Drawing for the job (mm, zero at the part's lowest x, y, z). A direction names the side the tool comes from. Give positions to 0.01 mm unless a question says otherwise; leave off trailing zeros. Loops run counter-clockwise (first coordinate to the right, second up) from the corner with the lowest first, then second, coordinate; pieces in that order, holes last. Notation, with made-up numbers: (-22.75, -4.75) - (5.25, -4.75) arc R7 cw to (5.25, 4.25) - close; hole circle Ø7 at (30.25, 66). An arc over 180 degrees is marked (long way). Return JSON: item names as keys, results as strings. Group by question number.
1) Slice it at C-C (x = 37). List the corners of the cut face in (y, z) (1 decimal).
2) Slice it at B-B (x = 22). List the corners of the cut face in (y, z) (1 decimal), and give its area (3 significant figures).
3) Drop flat-ended pins along their axis: pin 1 (6 mm diameter, centred on x = 43.5, y = 27, fed in from -Z); pin 2 (25 mm diameter, centred on x = 108.1, z = 56.41, fed in from +Y); pin 3 (4 mm diameter, centred on y = 18.5, z = 16.5, fed in from +X); pin 4 (1.5 mm diameter, centred on x = 50.5, z = 14, fed in from +Y). Give the stop position or say it passes through.
4) Drill centre lines: probe 1 along Z at (x, y) = (107, 55) (1 decimal); probe 2 along Y at (x, z) = (63.5, 47); probe 3 along Z at (x, y) = (48, 42) (1 decimal). Where is each one in solid material? Low to high. Write a range as from..to.
5) Mould opens along X. For the marked faces 4, 5, 6 and 7 say: released by +X, released by -X, zero draft, split by the parting line, or undercut.
6) 3-axis set-ups, long thin cutter, end or side, ignore diameter. For the marked faces 1, 2 and 3: which of +Z, -Z, +X, -X, +Y, -Y reach the whole face in a straight line?
7) Slice it at A-A (z = 58). List the corners of the cut face in (x, y) (1 decimal).
8) Slice it at D-D (z = 34). List the corners of the cut face in (x, y) (1 decimal).
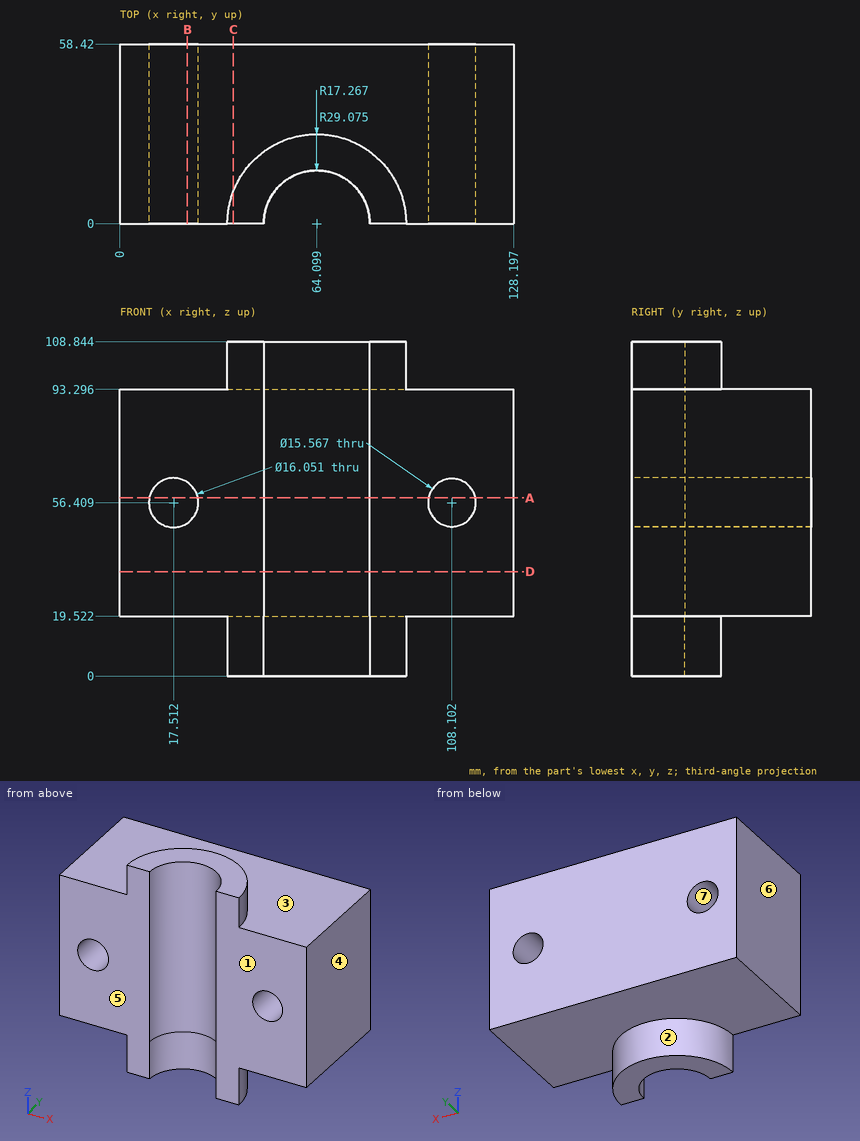
Results:
{
 "1": {"outline": "(0, 0) - (10.5, 0) - (10.5, 19.5) - (58.4, 19.5) - (58.4, 93.3) - (10.5, 93.3) - (10.5, 108.8) - (0, 108.8) - close"},
 "2": {"outline": "(0, 19.5) - (58.4, 19.5) - (58.4, 49.8) - (0, 49.8) - close; (0, 63.1) - (58.4, 63.1) - (58.4, 93.3) - (0, 93.3) - close", "area": "3,530 mm2"},
 "3": {"pin 1": "z = 19.52", "pin 2": "y = 58.42", "pin 3": "x = 88.04", "pin 4": "y = 26.08"},
 "4": {"probe 1": "19.5..48.7, 64.1..93.3", "probe 2": "17.26..58.42", "probe 3": "19.5..93.3"},
 "5": {"face 4": "released by +X", "face 5": "zero draft", "face 6": "released by -X", "face 7": "undercut"},
 "6": {"face 1": "+Z, -Z, +X, -X, -Y", "face 2": "-Z, +Y", "face 3": "+Z, +Y"},
 "7": {"outline": "(0, 0) - (9.6, 0) - (9.6, 58.4) - (0, 58.4) - close; (25.4, 0) - (46.8, 0) arc R17.3 cw to (81.4, 0) - (100.5, 0) - (100.5, 58.4) - (25.4, 58.4) - close; (115.7, 0) - (128.2, 0) - (128.2, 58.4) - (115.7, 58.4) - close"},
 "8": {"outline": "(0, 0) - (46.8, 0) arc R17.3 cw to (81.4, 0) - (128.2, 0) - (128.2, 58.4) - (0, 58.4) - close"}
}
